Source: CAD feature listing. Evaluate the final solid. Frame: model axes, mm. A direction names the side the tool comes from. Give positions to 0.01 mm unless a question says otherwise; leave off trailing zeros. Write each loop counter-clockwise with the first axis right and the second up, starting at its lowest first coordinate (ties: lowest second). Pieces come first, ordered by that corner, then holes. Notation, with made-up numbers: (-6.5, 75) -> (18.5, 75) arc R12 ccw to (18.5, 93) -> close; hole circle Ø2 at (-4.5, -15). An arc over 180 degrees is marked (long way). Answer as a JSON object with one key per item and string values. Group by question number.
Item 1: Section query C-C on z = 15. Return the cut outline in (x, y).
Item 2: Access query for faces 1 (the face through (60, -5, 15)), 2 (the face through (35, 0, 15)). Directions: +Z, -Z, +X, -X, +Y, -Y. A direction counts if a zero-diameter tool reaches every point of the face in a straight line with its end or side. Return the directions, or none.
Item 3: Section query A-A on x = 30. Return the cut outline in (y, z), plus the area to 3 significant figures.
Item 4: First-contact query: pin 1 Ø5.5 at (x, z) = (50, 15) entering from +Y; pin 2 Ø15 at (x, z) = (32, 10) entering from +Y; pin 3 Ø1 at (y, z) = (32, 10.5) entering from +X; pin 4 Ø5 at (y, z) = (4.5, 14) entering from +X. Flat tips, straight axial feed; report the tip coordinate or a pass-through.
Item 5: Section query D-D on z = 6.5. Return the cut outline in (x, y), plus the area to 3 significant figures.
Item 6: Pull-direction query (Z, two-part tool) for faces 3 (the face through (-5, 40, 15)), 4 (the face through (45.708, -5.07, 13.648)), 5 (the face through (12, -2, 0)); classes: pulls with the +Z half, pulls with the -Z half, needs draft (parallel to the pull), parting line crosses it, or undercut.
Item 7: Ray query, probe 1 along Z at (x, y) = (50, -4.75); probe 2 along Y at (x, z) = (-5.75, 15); probe 3 along Y at (x, z) = (12.5, 17.75). Return the intervals inside material, ascending. Write a range as from..to.
from build123d import *

# Parameters (mm, degrees)
BOSS_EXTRUDE1_DEPTH  = 30
M8_CLEARANCE_HOLE1_D = 9
M8_CLEARANCE_HOLE2_D = 9
FILLET1_R            = 10


with BuildPart() as part:
    # Sketch1 → Boss-Extrude1 (new body)
    with BuildSketch(Plane.XY):
        Polygon((0, 0), (0, 40), (-10, 40), (-10, -10), (10, -10), (60, -10), (60, 0), align=None)
    extrude(amount=BOSS_EXTRUDE1_DEPTH)

    # M8 Clearance Hole1 (through all)
    with Locations(Plane(origin=(0, 0, 0), x_dir=(0, 0, -1), z_dir=(1, 0, 0))):
        with Locations((-15, 27.5)):
            Hole(M8_CLEARANCE_HOLE1_D / 2)

    # M8 Clearance Hole2 (through all)
    with Locations(Plane(origin=(0, 0, 0), x_dir=(1, 0, 0), z_dir=(0, 1, 0))):
        with Locations((30, -15), (50, -15)):
            Hole(M8_CLEARANCE_HOLE2_D / 2)

    # Fillet1
    fillet1_edges = [part.edges().sort_by_distance(p)[0] for p in [
        (0, 0, 15),
    ]]
    fillet(fillet1_edges, radius=FILLET1_R)


solid = part.part
Worked answers:
{
 "1": {"outline": "(-10, -10) -> (25.5, -10) -> (25.5, 0) -> (10, 0) arc R10 cw to (0, 10) -> (0, 23) -> (-10, 23) -> close; (-10, 32) -> (0, 32) -> (0, 40) -> (-10, 40) -> close; (34.5, -10) -> (45.5, -10) -> (45.5, 0) -> (34.5, 0) -> close; (54.5, -10) -> (60, -10) -> (60, 0) -> (54.5, 0) -> close"},
 "2": {"face 1": "+Z, -Z, +X, +Y, -Y", "face 2": "+Z, -Z, +X, +Y"},
 "3": {"outline": "(-10, 0) -> (0, 0) -> (0, 10.5) -> (-10, 10.5) -> close; (-10, 19.5) -> (0, 19.5) -> (0, 30) -> (-10, 30) -> close", "area": "210 mm^2"},
 "4": {"pin 1": "through", "pin 2": "y = 0", "pin 3": "x = 0", "pin 4": "x = 4"},
 "5": {"outline": "(-10, -10) -> (60, -10) -> (60, 0) -> (10, 0) arc R10 cw to (0, 10) -> (0, 40) -> (-10, 40) -> close", "area": "1,120 mm^2"},
 "6": {"face 3": "needs draft", "face 4": "undercut", "face 5": "pulls with the -Z half"},
 "7": {"probe 1": "0..10.5, 19.5..30", "probe 2": "-10..23, 32..40", "probe 3": "-10..0"}
}
